from build123d import *

# Parameters (mm, degrees)
F0_W     = 54.61
F0_H     = 76.2
F0_R     = 11.43
F1_DEPTH = 76.2
F3_DEPTH = 88.9
F5_DEPTH = 101.6
F6_R     = 3.175


with BuildPart() as f1:
    # F0 (on Front) → F1 (new body, symmetric)
    with BuildSketch(Plane.XZ):
        with Locations((-14.605, 15.875)):
            Rectangle(F0_W, F0_H)
        Circle(F0_R, mode=Mode.SUBTRACT)
    extrude(amount=F1_DEPTH, both=True)

    # F2 (on Top) → F3 (intersect, symmetric)
    with BuildSketch(Plane.XY):
        with BuildLine():
            Line((12.7, 0), (-14.9225, 0))
            ThreePointArc((-14.9225, 0), (-22.1067048969, 2.9757951031), (-25.0825, 10.16))
            Line((-25.0825, 10.16), (-25.0825, 16.2052))
            ThreePointArc((-25.0825, 16.2052), (-30.0111606396, 28.1040393604), (-41.91, 33.0327))
            Line((-41.91, 33.0327), (-67.31, 33.0327))
            Line((-67.31, 33.0327), (-67.31, 31.4452))
            Line((-67.31, 31.4452), (-41.91, 31.4452))
            ThreePointArc((-41.91, 31.4452), (-31.1336926547, 26.9815073453), (-26.67, 16.2052))
            Line((-26.67, 16.2052), (-26.67, 10.16))
            ThreePointArc((-26.67, 10.16), (-23.229236912, 1.853263088), (-14.9225, -1.5875))
            Line((-14.9225, -1.5875), (12.7, -1.5875))
            Line((12.7, -1.5875), (12.7, 0))
        make_face()
    extrude(amount=F3_DEPTH, both=True, mode=Mode.INTERSECT)

    # F4 (on Right) → F5 (intersect, symmetric)
    with BuildSketch(Plane.YZ):
        Polygon((33.0327, 3.1664020477), (0, 14.605), (-1.5875, 14.605), (-1.5875, -22.225), (33.0327, -22.225), align=None)
    extrude(amount=F5_DEPTH, both=True, mode=Mode.INTERSECT)

    # F6
    f6_edges = [f1.edges().sort_by_distance(p)[0] for p in [
        (12.7, -0.79375, 14.605),
        (12.7, -0.79375, -22.225),
        (-41.91, 32.23895, 3.441263),
        (-41.91, 32.23895, -22.225),
    ]]
    fillet(f6_edges, radius=F6_R)


solid = f1.part
Can you work these out from the model? Positions are in its coordinate system, mm. A direction names the side the tool comes from. Give positions to 0.01 mm unless a question says otherwise; leave off trailing zeros. Loops run counter-clockwise (first coordinate to the right, second up) from the corner with the lowest first, then second, coordinate; pieces in that order, holes last. Notation, with made-up numbers: (39, 11.5) -> (82, 11.5) arc R19 ccw to (82, 34.5) -> close; hole circle Ø3 at (-38, 16). An arc over 180 degrees is marked (long way). Use one line per item in the form item = value.
1) If we section it at B-B (z = -16.5): Please give me the cut outline in (x, y) (1 decimal), plus the area to 3 significant figures.
Answers:
outline = (-41.9, 31.4) arc R15.2 cw to (-26.7, 16.2) -> (-26.7, 10.2) arc R11.7 ccw to (-14.9, -1.6) -> (12.7, -1.6) -> (12.7, 0) -> (-14.9, 0) arc R10.2 cw to (-25.1, 10.2) -> (-25.1, 16.2) arc R16.8 ccw to (-41.9, 33) -> close
area = 121 mm²
2) If we section it at D-D (y = 14): Please give me the cut outline in (x, z) (1 decimal), plus the area to 3 significant figures.
Answers:
outline = (-26.7, -22.2) -> (-25.1, -22.2) -> (-25.1, 9.8) -> (-26.7, 9.8) -> close
area = 50.8 mm²
3) If we section it at C-C (x = 6.5): Please give me the cut outline in (y, z) (1 decimal), plus the area to 3 significant figures.
Answers:
outline = (-1.6, -22.2) -> (0, -22.2) -> (0, -9.4) -> (-1.6, -9.4) -> close; (-1.6, 9.4) -> (0, 9.4) -> (0, 14.6) -> (-1.6, 14.6) -> close
area = 28.6 mm²
4) We'd pull the mould along Z, two halves only. Please class faces 1 (the face through (-25.891, 17.654, 8.492)), 2 (the face through (-41.005, 32.272, -21.27)), 3 (the face through (10.902, -0.783, 3.433)): released by +Z, released by -Z, zero draft, split by the parting line, or undercut.
Answers:
face_1 = released by +Z
face_2 = released by -Z
face_3 = undercut
5) I need wall thicknesses on line 1 along Z through (x, y) = (0, -0.85) (3 decimals); line 2 along Y through (x, z) = (-10.5, -14); line 3 along X through (y, z) = (12.5, 4.5). Which ranges of each line are inside material? Lowest first, please.
Answers:
line_1 = -22.225 to -11.43, 11.43 to 14.605
line_2 = -1.59 to 0
line_3 = -26.67 to -25.08
6) Will these pins go through, and if not, where does the flat tip stop? pin 1 (2 mm diameter, centred on y = 27, z = -5.5, fed in from +X); pin 2 (1.8 mm diameter, centred on y = 14, z = -10.5, fed in from -X); pin 3 (12 mm diameter, centred on x = -31.5, y = 21, fed in from -Z) (3 decimals); pin 4 (22 mm diameter, centred on x = 0, z = -12, fed in from +Y).
Answers:
pin_1 = -28.23
pin_2 = -26.67
pin_3 = -22.225
pin_4 = 0
7) For faces 4 (the face through (-25.082, 13, -5)), 5 (the face through (-26.67, 13, -5)), 6 (the face through (-1, -1.588, -12)), which set-ups out of +Z, -Z, +X, -X, +Y, -Y let a thin tool reach every point of the face, with its end or its side?
Answers:
face_4 = +Z, -Z, +X, +Y
face_5 = +Z, -Z, -X, -Y
face_6 = +Z, -Z, +X, -X, -Y
8) If we section it at A-A (x = 0): Please give me the cut outline in (y, z) (1 decimal).
Answers:
outline = (-1.6, -22.2) -> (0, -22.2) -> (0, -11.4) -> (-1.6, -11.4) -> close; (-1.6, 11.4) -> (0, 11.4) -> (0, 14.6) -> (-1.6, 14.6) -> close
